```python
from build123d import *

# Parameters (mm, degrees)
F0_W     = 54
F0_H     = 100
F1_DEPTH = 10
F2_R     = 4.602391418
F3_DEPTH = 2.3
F6_D     = 5
F6_DEPTH = 44
F6_TIP   = 1.5021515476


# Not quite as in the source:
# - a fillet or chamfer that OpenCascade refuses, or shapes differently, is made with other operations: its cross-section is extruded or revolved along the edge and cut away or added


with BuildPart() as f1:
    # F0 (on Front) → F1 (new body)
    with BuildSketch(Plane.XZ):
        with BuildLine():
            ThreePointArc((30, 56.5), (28.9748737342, 58.9748737342), (26.5, 60))
            Line((26.5, 60), (-26.5, 60))
            ThreePointArc((-26.5, 60), (-28.9748737342, 58.9748737342), (-30, 56.5))
            Line((-30, 56.5), (-30, -56.5))
            ThreePointArc((-30, -56.5), (-28.9748737342, -58.9748737342), (-26.5, -60))
            Line((-26.5, -60), (26.5, -60))
            ThreePointArc((26.5, -60), (28.9748737342, -58.9748737342), (30, -56.5))
            Line((30, -56.5), (30, 56.5))
        make_face()
        with Locations((-0.5, 6.5)):
            Rectangle(F0_W, F0_H, mode=Mode.SUBTRACT)
    extrude(amount=F1_DEPTH)

    # F2 (on face) → F3 (join)
    with BuildSketch(Plane.XZ.offset(10)):
        with Locations((0, -51.5322610736)):
            Circle(F2_R)
    extrude(amount=F3_DEPTH)

    # F4: fillet of radius 5.069848481 on 1 edges, made by hand

    # F4_s1 → F4_t2 (revolve, cut)
    with BuildSketch(Plane.XY.offset(-51.5322610736)):
        with BuildLine():
            ThreePointArc((4.602391418, -10), (2.7706699872, -11.6880700767), (0.356063238, -12.3))
            Line((0.356063238, -12.3), (4.602391418, -12.3))
            Line((4.602391418, -12.3), (4.602391418, -10))
        make_face()
    revolve(axis=Axis((0, -12.3, -51.5322610736), (0, -1, 0)), mode=Mode.SUBTRACT)

    # F6
    with Locations(Plane(origin=(0, 0, -60), x_dir=(1, 0, 0), z_dir=(0, 0, -1))):
        with Locations((14.8790339008, 5.0806454383)):
            Hole(F6_D / 2, depth=F6_DEPTH)
            with Locations((0, 0, -(F6_DEPTH + F6_TIP / 2))):  # 118° drill point
                Cone(0, F6_D / 2, F6_TIP, mode=Mode.SUBTRACT)


solid = f1.part
```
The model under review builds one solid part; all positions refer to its coordinate system, in mm. A direction names the side the tool comes from. Coordinates: 2 decimals unless noted, no trailing zeros. Write each loop counter-clockwise with the first axis right and the second up, starting at its lowest first coordinate (ties: lowest second). Pieces come first, ordered by that corner, then holes. Notation, with made-up numbers: (-5, 57) - (36, 57) arc R16 ccw to (36, 66) - close; hole circle Ø3 at (75.25, 37.5). An arc over 180 degrees is marked (long way). Answer in a Markdown table with one row per item. Add a question column.
Q1. Consider section A-A on x = 21.5. Give the boundary of the cut face in (y, z).
Q2. Consider section C-C on y = -6.25. Give the boundary of the cut face in (x, z).
Q3. Consider section D-D on x = 14.5. Give the boundary of the cut face in (y, z), then the cut area to 3 significant figures.
Q4. For faces 1 (the face through (26.5, -5, 6)), 2 (the face through (29, -4.93, 58.95)), list the 3-axis set-ups (+Z, -Z, +X, -X, +Y, -Y) from which the entire face can be reached by the end or side of a thin tool; tool diameter is ignored.
Q5. Draft analysis for pull direction Z (two halves, no side actions). For faces 3 (the face through (28.95, -4.93, -59)), 4 (the face through (17.377, -5.191, -51.634)), 5 (the face through (-1, -5, 56.5)), state which applies: +Z half, -Z half, draft (parallel to the pull), parting line (faces both ways), or undercut.
Q6. Consider section B-B on z = 27. Give the boundary of the cut face in (x, y).
Q7. To check wall thickness, follow line 1 along Z through (x, y) = (-10, -7.75); line 2 along X through (y, z) = (-8.5, 46.5); line 3 along Y through (x, z) = (22.5, -48). State the ranges of each line that lie inside material, in increasing order. Write a range as from..to.
Answers below:
| question | item | result |
|---|---|---|
| 1 | outline | (-10, -60) - (0, -60) - (0, -43.5) - (-10, -43.5) - close; (-10, 56.5) - (0, 56.5) - (0, 60) - (-10, 60) - close |
| 2 | outline | (-30, -56.5) arc R3.5 ccw to (-26.5, -60) - (12.67, -60) - (12.67, -43.5) - (-27.5, -43.5) - (-27.5, 56.5) - (26.5, 56.5) - (26.5, -43.5) - (17.09, -43.5) - (17.09, -60) - (26.5, -60) arc R3.5 ccw to (30, -56.5) - (30, 56.5) arc R3.5 ccw to (26.5, 60) - (-26.5, 60) arc R3.5 ccw to (-30, 56.5) - close |
| 3 | outline | (-10, -60) - (-7.55, -60) - (-7.55, -43.5) - (-10, -43.5) - close; (-10, 56.5) - (0, 56.5) - (0, 60) - (-10, 60) - close; (-2.61, -60) - (0, -60) - (0, -43.5) - (-2.61, -43.5) - close |
| 3 | area | 118 mm² |
| 4 | face 1 | +Y, -Y |
| 4 | face 2 | +Z, +X, +Y, -Y |
| 5 | face 3 | -Z half |
| 5 | face 4 | draft |
| 5 | face 5 | undercut |
| 6 | outline | (-30, -10) - (-27.5, -10) - (-27.5, 0) - (-30, 0) - close; (26.5, -10) - (30, -10) - (30, 0) - (26.5, 0) - close |
| 7 | line 1 | -60..-43.5, 56.5..60 |
| 7 | line 2 | -30..-27.5, 26.5..30 |
| 7 | line 3 | -10..0 |
